Could you check a few things on this drawing? It's one solid part, dimensions in mm from its lowest x, y, z. Give positions to 0.01 mm unless a question says otherwise; leave off trailing zeros. Order: outer loops, then holes, each group sorted by start corner. A loop starts at its lowest first (then second) coordinate and runs counter-clockwise, first axis right, second up. Notation, with made-up numbers: (-9, 9.25) - (49, 9.25) arc R34 ccw to (49, 40.25) - close; hole circle Ø5 at (54, 65.5). An arc over 180 degrees is marked (long way). Put each result on its own line as item: value.
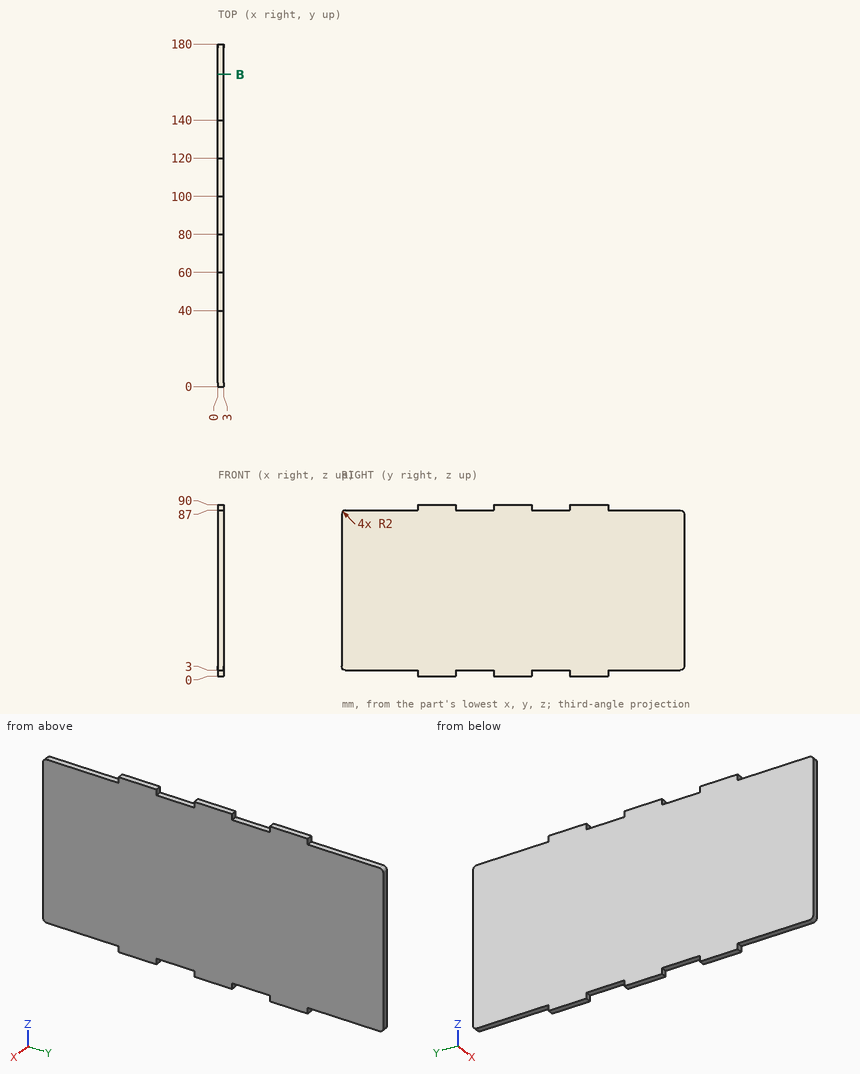
1) If I drill on line 1 (Z direction, x = 0.7, y = 149), over which ranges is the centre line in solid material (lowest first)? Write a range as [from, to].
Filled in:
line 1: z = [3, 87]
2) I'm going to push flat-ended pins straight in: pin 1 (0.9 mm diameter, centred on x = 2, z = 1.5, fed in from -Y); pin 2 (1.5 mm diameter, centred on x = 2, z = 1, fed in from +Y); pin 3 (10 mm diameter, centred on y = 120, z = 79.5, fed in from -X); pin 4 (1.5 mm diameter, centred on x = 1.5, y = 70.5, fed in from -Z). Where does each tip first touch, or does it pass through?
Filled in:
pin 1: stops at y = 40
pin 2: stops at y = 140
pin 3: stops at x = 0
pin 4: stops at z = 3
3) Suppose I cut it at B-B, the plane y = 164. List the corners of the cut face in (x, z) for me.
Filled in:
outline: (0, 3) - (3, 3) - (3, 87) - (0, 87) - close
